Autodesk Inventor part; units mm, degrees
ref_plane "YZ Plane" through (0, 0, 0) normal (1, 0, 0) x (0, 1, 0)
ref_plane "XZ Plane" through (0, 0, 0) normal (0, 1, 0) x (-1, 0, 0)
ref_plane "XY Plane" through (0, 0, 0) normal (0, 0, 1) x (1, 0, 0)
sketch "Skizze1" plane through (0, 0, 0) normal (0, 1, 0) x (-1, 0, 0)
  line L0 (25, -25) -> (-25, -25)
  line L1 (-25, -25) -> (-25, 25)
  line L2 (-25, 25) -> (25, 25)
  line L3 (25, 25) -> (25, -25)
  line L4 (0, -70.9121) -> (0, 70.9121)
  line L5 (0, -25) -> (-70.4769, -50.6515)
  line L6 (-70.4769, -50.6515) -> (-77.3173, -31.8577)
  line L7 (-77.3173, -31.8577) -> (-42.0428, -19.0188)
  line L8 (842.0086, 0) -> (-811.3812, 0)
  line L9 (0, -25) -> (70.4769, -50.6515)
  line L10 (70.4769, -50.6515) -> (77.3173, -31.8577)
  line L11 (77.3173, -31.8577) -> (42.0428, -19.0188)
  line L12 (-842.0086, 0) -> (811.3812, 0)
  line L13 (0, 25) -> (-70.4769, 50.6515)
  line L14 (-70.4769, 50.6515) -> (-77.3173, 31.8577)
  line L15 (-77.3173, 31.8577) -> (-42.0428, 19.0188)
  line L16 (77.3173, 31.8577) -> (42.0428, 19.0188)
  line L17 (0, 25) -> (70.4769, 50.6515)
  line L18 (70.4769, 50.6515) -> (77.3173, 31.8577)
  line L19 (-42.0428, -19.0188) -> (-25, 0)
  line L20 (42.0428, -19.0188) -> (25, 0)
  line L21 (-42.0428, 19.0188) -> (-25, 0)
  line L22 (42.0428, 19.0188) -> (25, 0)
  point P0 (0, 0)
  dimension "d0" = 50
  dimension "d1" = 50
  dimension "d3" = 75
  dimension "d6" = 20
  dimension "d7" = 20
  dimension "d8" = 90
  dimension "d12" = 41.864
extrude "Extrusion1" add sketch "Skizze1" along normal blind 2
sketch "Skizze2" plane through (0, 2, 0) normal (0, 1, 0) x (1, 0, 0)
  circle A0 centre (-66.8909, 42.9612) radius 1.6
  line L0 (0, 25) -> (-70.4769, 50.6515)
  line L1 (-70.4769, 50.6515) -> (-77.3173, 31.8577)
  circle A1 centre (-69.6271, 35.4437) radius 1.6
  line L2 (-77.3173, 31.8577) -> (-42.0428, 19.0188)
  line L3 (0, 70.9121) -> (0, -70.9121)
  line L4 (108.2443, 0) -> (-108.2443, 0)
  circle A2 centre (66.8909, 42.9612) radius 1.6
  circle A3 centre (69.6271, 35.4437) radius 1.6
  circle A4 centre (-66.8909, -42.9612) radius 1.6
  circle A5 centre (-69.6271, -35.4437) radius 1.6
  circle A6 centre (66.8909, -42.9612) radius 1.6
  circle A7 centre (69.6271, -35.4437) radius 1.6
  point P0 (0, 0)
  dimension "d15" = 3.2
  dimension "d16" = 6
  dimension "d17" = 6
  dimension "d18" = 3.2
  dimension "d19" = 6
  dimension "d20" = 6
extrude "Extrusion2" cut sketch "Skizze2" against normal up to surface (2 mm away)
sketch "Skizze3" plane through (0, 2, 0) normal (0, 1, 0) x (1, 0, 0)
  circle A0 centre (-18, 10) radius 1.6
  line L0 (0, 70.9121) -> (0, -70.9121)
  line L1 (108.2443, 0) -> (-108.2443, 0)
  circle A1 centre (-18, -10) radius 1.6
  circle A2 centre (18, 10) radius 1.6
  circle A3 centre (18, -10) radius 1.6
  point P0 (0, 0)
  dimension "d23" = 3.2
  dimension "d24" = 18
  dimension "d25" = 10
extrude "Extrusion3" cut sketch "Skizze3" against normal up to surface (2 mm away)
properties part number "_3D-Druck"
Check sheet for the modelled part. Datum: model origin and axes. Units: mm. A direction names the side the tool comes from. Round coordinates to 2 decimals unless told otherwise and drop trailing zeros. Order: outer loops, then holes, each group sorted by start corner. A loop starts at its lowest first (then second) coordinate and runs counter-clockwise, first axis right, second up. Notation, with made-up numbers: (68, 13.5) -> (125, 13.5) arc R26 cw to (125, 39.5) -> close; hole circle Ø11 at (1.5, -33.75). An arc over 180 degrees is marked (long way). Use CSV: the item, a comma, the result in double quotes.
(1) Cross-section at B-B (z = 28.5). Record the boundary of the cut face in (x, y), and give its area (3 significant figures).
Worked out:
outline,"(-68.09, 0) -> (-9.62, 0) -> (-9.62, 2) -> (-68.09, 2) -> close; (9.62, 0) -> (68.09, 0) -> (68.09, 2) -> (9.62, 2) -> close"
area,"234 mm²"
(2) Cross-section at D-D (x = -57). Record the boundary of the cut face in (y, z).
Worked out:
outline,"(0, -45.75) -> (2, -45.75) -> (2, -24.46) -> (0, -24.46) -> close; (0, 24.46) -> (2, 24.46) -> (2, 45.75) -> (0, 45.75) -> close"
(3) Depth check by flat-ended pin: pin 1 (1 mm diameter, centred on y = 1.5, z = -4.5, fed in from -X). Enter the tip coordinate at first touch or a pass-through.
Worked out:
pin 1,"x = -29.48"
(4) Draft check along Z on faces 5 (the face through (16.73, 1.01, -9.03)), 6 (the face through (-73.849, 0.986, -41.386)), 7 (the face through (59.93, 0.99, 25.53)), 8 (the face through (1, 2, 1)). Enter one of: pulls with the +Z half, pulls with the -Z half, needs draft (parallel to the pull), parting line crosses it, or undercut.
Worked out:
face 5,"undercut"
face 6,"pulls with the -Z half"
face 7,"undercut"
face 8,"needs draft"
(5) Material ranges on line 1 along X through (y, z) = (1.3, -10); line 2 along Z through (x, y) = (-63.5, 0.85); line 3 along Z through (x, y) = (47, 1.75), recorded low to high. Write a range as from..to.
Worked out:
line 1,"-33.96..-19.6, -16.4..16.4, 19.6..33.96"
line 2,"-48.11..-26.83, 26.83..48.11"
line 3,"-42.11..-20.82, 20.82..42.11"
(6) Cross-section at C-C (y = 0.6). Count the separate pieces of the cut face and the enclosed holes in it, and give its area (3 significant figures).
Worked out:
separate pieces,"1"
enclosed holes,"12"
area,"7,460 mm²"
(7) Tool access check on faces 1 (the face through (59.93, 0.99, -25.53)), 2 (the face through (68.37, 1.01, 43.57)), 3 (the face through (34.75, 0.99, 37.65)), 4 (the face through (-33.6, 1, 9.6)). Record the directions out of +Z, -Z, +X, -X, +Y, -Y that give a thin tool (end or side, any length) a straight path to the whole face; none if there is none.
Worked out:
face 1,"+X, +Y, -Y"
face 2,"+Y, -Y"
face 3,"+Z, +Y, -Y"
face 4,"-X, +Y, -Y"
(8) Cross-section at A-A (x = -18). Record the boundary of the cut face in (y, z), and give its area (3 significant figures).
Worked out:
outline,"(0, -31.55) -> (2, -31.55) -> (2, -11.6) -> (0, -11.6) -> close; (0, -8.4) -> (2, -8.4) -> (2, 8.4) -> (0, 8.4) -> close; (0, 11.6) -> (2, 11.6) -> (2, 31.55) -> (0, 31.55) -> close"
area,"113 mm²"
